```python
from build123d import *

# Parameters (mm, degrees)
F0_W         = 40
F0_H         = 40
F1_DEPTH     = 20
F3_DEPTH     = 18
F4_DEPTH     = 8
F5_R         = 48.402363322
F6_DEPTH     = 25
F7_R         = 8
F8_DEPTH     = 47.3578016938
F11_DEPTH    = 37.5
F12_DEPTH    = 12.05
F13_R        = 3.85
F14_DEPTH    = 2
F15_DEPTH    = 25
F16_R        = 7
F17_DEPTH    = 13
F18_DEPTH    = 18.5
F19_R        = 1
F20_R        = 11.2
F20_R_2      = 9.2
F21_DEPTH    = 1
F22_T1_DEPTH = 26.5487978578
F22_T3_DEPTH = 53.3816135878
F22_T5_DEPTH = 53.3816135878
F22_T7_DEPTH = 26.5487978578
F22_T9_DEPTH = 42.6013795348


# Not quite as in the source:
# - a fillet or chamfer that OpenCascade refuses, or shapes differently, is made with other operations: its cross-section is extruded or revolved along the edge and cut away or added


with BuildPart() as f1:
    # F0 (on Top) → F1 (new body)
    with BuildSketch(Plane.XY):
        Rectangle(F0_W, F0_H)
    extrude(amount=F1_DEPTH)

    # F3 (add): a face of the model
    f3_faces = [f1.faces().sort_by_distance(p)[0] for p in [
        (0, 0, 0),
    ]]
    extrude(f3_faces, amount=F3_DEPTH)

    # F4 (add): a face of the model
    f4_faces = [f1.faces().sort_by_distance(p)[0] for p in [
        (0, 0, 20),
    ]]
    extrude(f4_faces, amount=F4_DEPTH)

    # F5 (on 3pt) → F6 (cut)
    with BuildSketch(Plane(origin=(-6.6666666667, 6.6666666667, 13.3333333333), x_dir=(0.9128709292, 0.1825741858, 0.3651483717), z_dir=(-0.4082482905, 0.4082482905, 0.8164965809))):
        with Locations((2.3868493736, -7.4885585345)):
            Circle(F5_R)
    extrude(amount=F6_DEPTH, mode=Mode.SUBTRACT)

    # F7 (on face) → F8 (cut, through all)
    with BuildSketch(Plane(origin=(-6.6666666667, 6.6666666667, 13.3333333333), x_dir=(0.9128709292, 0.1825741858, 0.3651483717), z_dir=(-0.4082482905, 0.4082482905, 0.8164965809))):
        with Locations((5.3147843089, -6.5092548249)):
            Circle(F7_R)
    extrude(amount=-F8_DEPTH, mode=Mode.SUBTRACT)

    # F10 (on offset) → F11 (cut, symmetric)
    with BuildSketch(Plane(origin=(9.6632649519, -9.6632649519, -19.3265299038), x_dir=(0.9128709292, 0.1825741858, 0.3651483717), z_dir=(-0.4082482905, 0.4082482905, 0.8164965809))):
        Polygon((16.712234718, -4.6568354596), (9.4092672846, 4.2874364504), (-1.9881831245, 2.4350170851), (-6.0826661002, -8.3616741902), (1.2203013332, -17.3059461002), align=None)
        Polygon((12.6177517423, -15.4535267349), (16.712234718, -4.6568354596), (1.2203013332, -17.3059461002), align=None)
    extrude(amount=F11_DEPTH, both=True, mode=Mode.SUBTRACT)

    # F10 (on offset) → F12 (cut)
    with BuildSketch(Plane(origin=(9.6632649519, -9.6632649519, -19.3265299038), x_dir=(0.9128709292, 0.1825741858, 0.3651483717), z_dir=(-0.4082482905, 0.4082482905, 0.8164965809))):
        Polygon((44.0977028976, 17.7033056762), (16.712234718, -4.6568354596), (12.6177517423, -15.4535267349), (1.2203013332, -17.3059461002), (-18.4589771374, -33.3740096866), (-1.5124044388, -54.1292376868), (61.0442755962, -3.051922324), align=None)
    extrude(amount=F12_DEPTH, mode=Mode.SUBTRACT)

    # F13 (on face) → F14 (join)
    with BuildSketch(Plane(origin=(0, 0, -18), x_dir=(1, 0, 0), z_dir=(0, 0, -1))):
        with Locations((-13.5, 13.5)):
            Circle(F13_R)
        with Locations((-13.5, -13.5)):
            Circle(F13_R)
        with Locations((13.5, -13.5)):
            Circle(F13_R)
    extrude(amount=F14_DEPTH)

    # F13 (on face) → F15 (cut)
    with BuildSketch(Plane(origin=(0, 0, -18), x_dir=(1, 0, 0), z_dir=(0, 0, -1))):
        with BuildLine():
            ThreePointArc((0.2498865688, 4.1424698795), (0, 4.4), (-0.2498865688, 4.1424698795))
            ThreePointArc((-0.2498865688, 4.1424698795), (-3.5940054257, 2.075), (-3.7124274345, -1.8548268231))
            ThreePointArc((-3.7124274345, -1.8548268231), (-3.8105117767, -2.2), (-3.4625408657, -2.2876430564))
            ThreePointArc((-3.4625408657, -2.2876430564), (0, -4.15), (3.4625408657, -2.2876430564))
            ThreePointArc((3.4625408657, -2.2876430564), (3.8105117767, -2.2), (3.7124274345, -1.8548268231))
            ThreePointArc((3.7124274345, -1.8548268231), (3.5940054257, 2.075), (0.2498865688, 4.1424698795))
        make_face()
    extrude(amount=-F15_DEPTH, mode=Mode.SUBTRACT)

    # F16 (on Top) → F17 (cut)
    with BuildSketch(Plane.XY):
        Circle(F16_R)
    extrude(amount=-F17_DEPTH, mode=Mode.SUBTRACT)

    # F16 (on Top) → F18 (cut)
    with BuildSketch(Plane.XY):
        Circle(F16_R)
    extrude(amount=F18_DEPTH, mode=Mode.SUBTRACT)

    # F19
    f19_edges = [f1.edges().sort_by_distance(p)[0] for p in [
        (-17.35, 13.5, -20),
        (-17.35, -13.5, -20),
        (9.65, 13.5, -20),
    ]]
    fillet(f19_edges, radius=F19_R)

    # F20 (on face) → F21 (join)
    with BuildSketch(Plane(origin=(-6.6666666667, 6.6666666667, 13.3333333333), x_dir=(0.9128709292, 0.1825741858, 0.3651483717), z_dir=(-0.4082482905, 0.4082482905, 0.8164965809))):
        Polygon((2.9211869734, -30.410524494), (29.2118697336, -8.94427191), (29.2118697336, 8.94427191), (-14.6059348668, 17.88854382), (-14.6059348668, -26.83281573), align=None)
        Polygon((27.2118697336, -7.9952761744), (2.3913648452, -28.2611335526), (-12.6059348668, -25.1998225681), (-12.6059348668, 15.4390540772), (27.2118697336, 7.3112787481), align=None, mode=Mode.SUBTRACT)
        with Locations((5.3147843089, -6.5092548249)):
            Circle(F20_R)
        with Locations((5.3147843089, -6.5092548249)):
            Circle(F20_R_2, mode=Mode.SUBTRACT)
    extrude(amount=F21_DEPTH)

    # F22: fillet of radius 2 on 5 edges, made by hand

    # F22_s2 → F22_t1 (cut)
    with BuildSketch(Plane(origin=(-11.8729833462, 0, -5.9364916731), x_dir=(0, 1, 0), z_dir=(0.894427191, 0, 0.4472135955))):
        with BuildLine():
            ThreePointArc((-20, 26.83281573), (-19.0328736084, 27.2022251402), (-18.0106128795, 27.038579878))
            Line((-18.0106128795, 27.038579878), (-17.9942829478, 27.0750947152))
            Line((-17.9942829478, 27.0750947152), (-19.5754217779, 27.7822014963))
            Line((-19.5754217779, 27.7822014963), (-19.6282665467, 27.7620165908))
            ThreePointArc((-19.6282665467, 27.7620165908), (-19.8323906919, 27.3055811262), (-20.0234578108, 26.8652152842))
            Line((-20.0234578108, 26.8652152842), (-20, 26.83281573))
        make_face()
    extrude(amount=F22_T1_DEPTH, mode=Mode.SUBTRACT)

    # F22_s4 → F22_t3 (cut)
    with BuildSketch(Plane(origin=(0, 19.8729833462, -9.9364916731), x_dir=(1, 0, 0), z_dir=(0, -0.894427191, 0.4472135955))):
        with BuildLine():
            ThreePointArc((-20, 8.94427191), (-19.6305905898, 9.9113983016), (-18.8271094604, 10.5642496204))
            Line((-18.8271094604, 10.5642496204), (-18.843439392, 10.6007644575))
            Line((-18.843439392, 10.6007644575), (-20.4245782221, 9.8936576763))
            Line((-20.4245782221, 9.8936576763), (-20.4447631276, 9.8408129076))
            ThreePointArc((-20.4447631276, 9.8408129076), (-20.2406389824, 9.384377443), (-20.0397877424, 8.948387193))
            Line((-20.0397877424, 8.948387193), (-20, 8.94427191))
        make_face()
    extrude(amount=F22_T3_DEPTH, mode=Mode.SUBTRACT)

    # F22_s6 → F22_t5 (cut)
    with BuildSketch(Plane(origin=(27.8729833462, 0, 13.9364916731), x_dir=(0, 1, 0), z_dir=(-0.894427191, 0, -0.4472135955))):
        with BuildLine():
            ThreePointArc((20, -8.94427191), (19.6305905898, -9.9113983016), (18.8271094604, -10.5642496204))
            Line((18.8271094604, -10.5642496204), (18.843439392, -10.6007644575))
            Line((18.843439392, -10.6007644575), (20.4245782221, -9.8936576763))
            Line((20.4245782221, -9.8936576763), (20.4447631276, -9.8408129076))
            ThreePointArc((20.4447631276, -9.8408129076), (20.2406389824, -9.384377443), (20.0397877424, -8.948387193))
            Line((20.0397877424, -8.948387193), (20, -8.94427191))
        make_face()
    extrude(amount=F22_T5_DEPTH, mode=Mode.SUBTRACT)

    # F22_s8 → F22_t7 (cut)
    with BuildSketch(Plane(origin=(0, -11.8729833462, 5.9364916731), x_dir=(1, 0, 0), z_dir=(0, 0.894427191, -0.4472135955))):
        with BuildLine():
            ThreePointArc((20, -26.83281573), (19.0328736084, -27.2022251402), (18.0106128795, -27.038579878))
            Line((18.0106128795, -27.038579878), (17.9942829478, -27.0750947152))
            Line((17.9942829478, -27.0750947152), (19.5754217779, -27.7822014963))
            Line((19.5754217779, -27.7822014963), (19.6282665467, -27.7620165908))
            ThreePointArc((19.6282665467, -27.7620165908), (19.8323906919, -27.3055811262), (20.0234578108, -26.8652152842))
            Line((20.0234578108, -26.8652152842), (20, -26.83281573))
        make_face()
    extrude(amount=F22_T7_DEPTH, mode=Mode.SUBTRACT)

    # F22_s10 → F22_t9 (cut)
    with BuildSketch(Plane(origin=(-15.0618621785, -15.0618621785, 0), x_dir=(0, 0, 1), z_dir=(0.7071067812, 0.7071067812, 0))):
        with BuildLine():
            ThreePointArc((27.8164965809, 9.3221446674), (28.1750672506, 10.2933417867), (28, 11.313708499))
            Line((28, 11.313708499), (28.0363299316, 11.3304457648))
            ThreePointArc((28.0363299316, 11.3304457648), (28.4313423012, 11.0576932276), (28.8395905917, 10.769018093))
            Line((28.8395905917, 10.769018093), (28.8491564442, 10.713264219))
            Line((28.8491564442, 10.713264219), (27.8491564442, 9.2990506567))
            Line((27.8491564442, 9.2990506567), (27.8164965809, 9.3221446674))
        make_face()
    extrude(amount=F22_T9_DEPTH, mode=Mode.SUBTRACT)


solid = f1.part
```
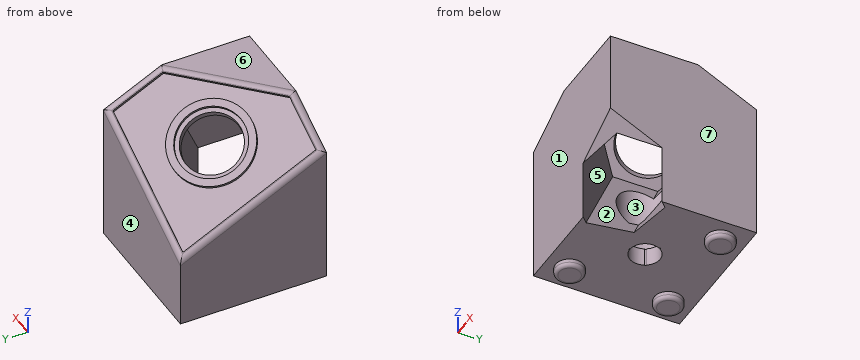
The listing builds one solid part. Answer for the finished solid, in the listing's coordinates (mm). Face numbers are marked on the shaded views. A direction names the side the tool comes from. Coordinates: 2 decimals unless noted, no trailing zeros. Write each loop counter-clockwise with the first axis right and the second up, starting at its lowest first coordinate (ties: lowest second). Pieces come first, ordered by that corner, then holes. Notation, with made-up numbers: M -27.75,-13.75 L -2.75,-13.75 A28 cw -2.75,19.25 Z; hole C 66,37.5 d1. An arc over 180 degrees is marked long. Use a Markdown table: item, result. Add a question column.
1. Given P1, Ø10, axis at x = -7, y = -2, coming from the -Z side; P2, Ø4, axis at x = -7.5, y = -11, coming from the +Z side; P3, Ø1.5, axis at x = 13.5, y = -14, coming from the +Z side, each flat-ended and moving along its own axis, determine where each tip first touches the part or whether it passes through.
2. Which of the six approach directions +Z, -Z, +X, -X, +Y, -Y give full straight-line access (tool end or side, diameter ignored) to the marked faces 5, 6 and 7?
3. Straight lines are drawn through the part: line 1 along X through (y, z) = (-0.5, 12); line 2 along Z through (x, y) = (18, -2); line 3 along Z through (x, y) = (7, 7). For each, find the intervals that lie inside material, in ascending order. Write a range as [from, to].
4. For a pull along Y with two mould halves and no side action, classify the marked faces 1, 2, 3 and 4 as +Y half, -Y half, draft (parallel to the pull), parting line (faces both ways), or undercut.
5. Section B-B (z = -2) is taken. Give the vertices of the cut face in (x, y).
6. Section C-C (z = -10) is taken. Give the vertices of the cut face in (x, y), plus the area to 3 significant figures.
Data:
| question | item | result |
|---|---|---|
| 1 | P1 | stops at z = -18 |
| 1 | P2 | stops at z = 23.16 |
| 1 | P3 | stops at z = 28 |
| 2 | face 5 | none |
| 2 | face 6 | +Z, +X, -Y |
| 2 | face 7 | +Z, -Z, +X, +Y, -Y |
| 3 | line 1 | x = [-18.94, -18.51], [-16.5, -10.3], [13.13, 20] |
| 3 | line 2 | z = [-18, 28] |
| 3 | line 3 | z = [-18, 4.45], [16.94, 21.22] |
| 4 | face 1 | -Y half |
| 4 | face 2 | undercut |
| 4 | face 3 | undercut |
| 4 | face 4 | +Y half |
| 5 | outline | M -20,-20 L 5.86,-20 L -3.79,-10.35 L -3.1,-6.28 A7 cw long 6.28,3.1 L 10.35,3.79 L 20,-5.86 L 20,20 L -20,20 Z |
| 6 | outline | M -20,-20 L 5.86,-20 L 0.21,-14.35 L 1.5,-6.84 A7 cw long 6.84,-1.5 L 14.35,-0.21 L 20,-5.86 L 20,20 L -20,20 Z |
| 6 | area | 1,130 mm2 |
